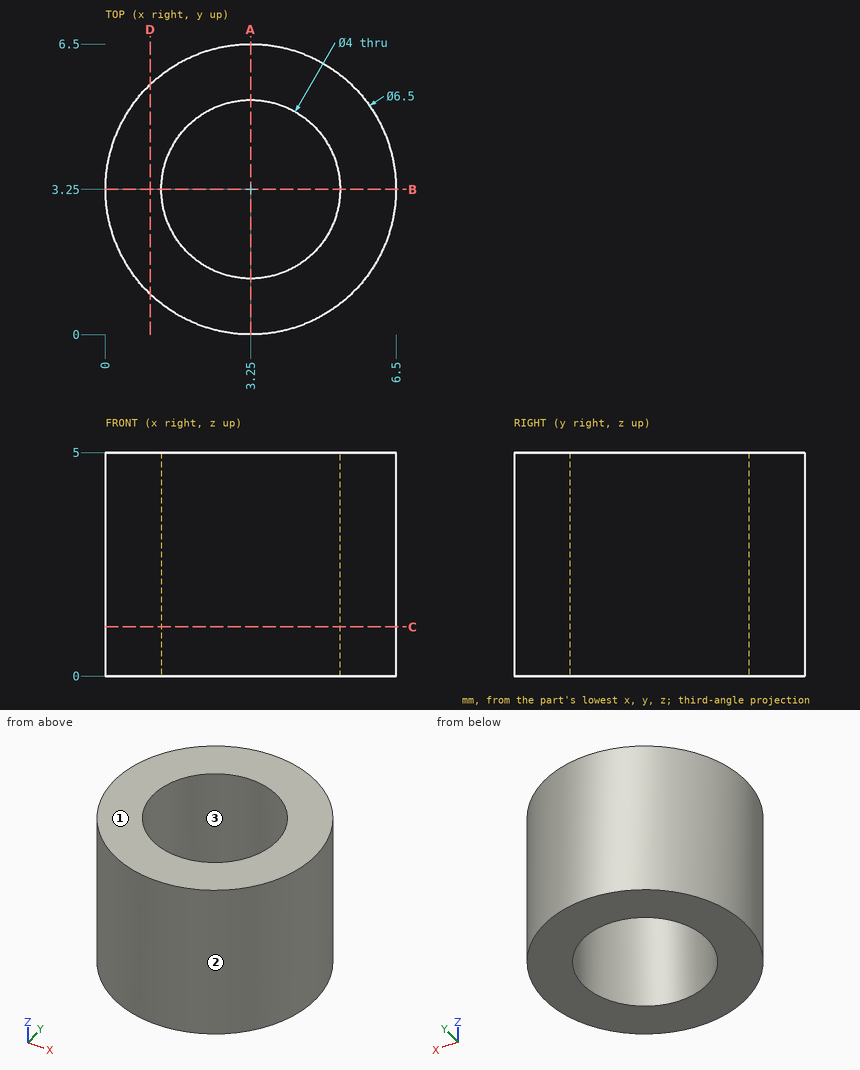
Check sheet for the drawn part. Datum: minimum x, y, z corner. Units: mm. Round coordinates to 2 decimals unless told otherwise and drop trailing zeros. Order: outer loops, then holes, each group sorted by start corner. A loop starts at its lowest first (then second) coordinate and runs counter-clockwise, first axis right, second up.
(1) Draft check along Y on the marked faces 1, 2 and 3. Enter one of: pulls with the +Y half, pulls with the -Y half, needs draft (parallel to the pull), parting line crosses it, or undercut.
(2) Scan lines: probe 1 along Y at (x, z) = (3.25, 1.1); probe 2 along Y at (x, z) = (2.5, 1.6). Record each from-to range of solid material in increasing order.
(3) Go/stop test with flat-tipped pins: P1, Ø1, axis at x = 1.5, z = 1, coming from the -Y side; P2, Ø1, axis at y = 1.5, z = 1.5, coming from the +X side; P3, Ø3.5, axis at x = 3.25, y = 3.25, coming from the -Z side. Record where each tip stops, or that it passes through.
(4) Cross-section at A-A, the plane x = 3.25. Enter the section's corners in (y, z).
(5) Cross-section at D-D, the plane x = 1. Enter the section's corners in (y, z), and give its area (3 significant figures).
(6) Cross-section at C-C, the plane z = 1.1. Enter the section's corners in (x, y).
Check sheet entries:
1. face 1: needs draft
1. face 2: parting line crosses it
1. face 3: undercut
2. probe 1: y = 0 to 1.25, 5.25 to 6.5
2. probe 2: y = 0.09 to 1.4, 5.1 to 6.41
3. P1: stops at y = 0.25
3. P2: stops at x = 6.25
3. P3: passes through
4. outline: (0, 0) - (1.25, 0) - (1.25, 5) - (0, 5) - close; (5.25, 0) - (6.5, 0) - (6.5, 5) - (5.25, 5) - close
5. outline: (0.9, 0) - (5.6, 0) - (5.6, 5) - (0.9, 5) - close
5. area: 23.5 mm2
6. outline: circle Ø6.5 at (3.25, 3.25); hole circle Ø4 at (3.25, 3.25)
